from build123d import *

# Parameters (mm, degrees)
PAD_DEPTH = 5
FILLET_R  = 1


with BuildPart() as part:
    # Sketch → Pad (new body)
    with BuildSketch(Plane.XZ):
        with BuildLine():
            Line((-8, 5.95), (-8, -6.95))
            Line((-8, -6.95), (-5.7, -6.95))
            Line((-5.7, -6.95), (-5.7, -10.75))
            Line((-5.7, -10.75), (-8.5, -10.75))
            ThreePointArc((-10.5, -8.75), (-9.914214, -10.164214), (-8.5, -10.75))
            Line((-10.5, -8.75), (-10.5, 7.45))
            ThreePointArc((-8.5, 9.45), (-9.914214, 8.864214), (-10.5, 7.45))
            Line((-8.5, 9.45), (8.5, 9.45))
            ThreePointArc((10.5, 7.45), (9.914214, 8.864214), (8.5, 9.45))
            Line((10.5, 7.45), (10.5, -8.75))
            ThreePointArc((8.5, -10.75), (9.914214, -10.164214), (10.5, -8.75))
            Line((8.5, -10.75), (5.7, -10.75))
            Line((5.7, -10.75), (5.7, -6.95))
            Line((5.7, -6.95), (8, -6.95))
            Line((8, -6.95), (8, 5.95))
            ThreePointArc((8, 5.95), (7.707107, 6.657107), (7, 6.95))
            Line((7, 6.95), (-7, 6.95))
            ThreePointArc((-7, 6.95), (-7.707107, 6.657107), (-8, 5.95))
        make_face()
    extrude(amount=PAD_DEPTH)

    # Fillet
    fillet_edges = [part.edges().sort_by_distance(p)[0] for p in [
        (-6.85, -5, -6.95),
        (-8, -5, -0.5),
        (-5.7, -2.5, -6.95),
        (-5.7, -5, -8.85),
        (-5.7, -2.5, -10.75),
        (-10.5, -5, -0.65),
        (-8, 0, -0.5),
        (-6.85, 0, -6.95),
        (-5.7, 0, -8.85),
        (0, 0, 9.45),
        (5.7, -5, -8.85),
        (5.7, -2.5, -10.75),
        (5.7, 0, -8.85),
        (5.7, -2.5, -6.95),
        (6.85, -5, -6.95),
        (7.1, -5, -10.75),
        (10.5, -5, -0.65),
        (8, -5, -0.5),
        (8, 0, -0.5),
        (-10.5, 0, -0.65),
        (0, -5, 9.45),
        (10.5, 0, -0.65),
        (6.85, 0, -6.95),
    ]]
    fillet(fillet_edges, radius=FILLET_R)


solid = part.part
Design review of the part built by this model. Coordinates are the model's own, in mm. A direction names the side the tool comes from. Round coordinates to 2 decimals unless told otherwise and drop trailing zeros. Write each loop counter-clockwise with the first axis right and the second up, starting at its lowest first coordinate (ties: lowest second). Pieces come first, ordered by that corner, then holes. Notation, with made-up numbers: (55.5, 66) - (111.5, 66) arc R20 cw to (111.5, 72) - close; hole circle Ø2 at (48.25, 0.5). An arc over 180 degrees is marked (long way). Return JSON: item names as keys, results as strings. Group by question number.
Item 1: We need section D-D on z = -7.5. Write out the cut boundary in (x, y).
Item 2: We need section B-B on y = -1.65. Write out the cut boundary in (x, z).
Item 3: Insertion check: P1, Ø0.9, axis at x = 1.5, y = -2, coming from the -Z side; P2, Ø0.9, axis at y = -2, z = -9, coming from the +X side; P3, Ø2, axis at x = -6.5, z = -6.5, coming from the -Y side. Each pin has a flat end and moves straight along its axis. Give the tip position at first contact, or say it passes through.
Item 4: We need section A-A on z = -1. Write out the cut boundary in (x, y).
Item 5: We need section C-C on x = 2.5. Write out the cut boundary in (y, z), and give its area (3 significant figures).
Item 6: For probe 1 along X at (y, z) = (-3.4, 5.75); probe 2 along X at (y, z) = (-1.15, -8.5); probe 3 along Z at (x, y) = (-3.25, -2.1), list the stretches that pass through material, from the lowest coordinate up. Write a range as [from, to].
Item 7: Machinability: for faces 1 (the face through (-0.098, -0.301, 7.235)), 2 (the face through (-7.699, -2.479, 6.665)), 3 (the face through (8.285, -4.699, -0.903)), 4 (the face through (-5.985, -4.699, -8.863)), which of the approach directions +Z, -Z, +X, -X, +Y, -Y give a long, thin tool a straight path to every point of the face, cutting with its end or side? Answer none if there is none.
Item 8: The part is to be moulded in two halves that separate along Z. For faces 5 (the face through (10.215, -4.699, -0.763)), 6 (the face through (5.985, -2.521, -7.251)), 7 (the face through (7.587, -0.301, -10.465)), say which applies: pulls with the +Z half, pulls with the -Z half, needs draft (parallel to the pull), parting line crosses it, or undercut.
Model answer:
{
 "1": {"outline": "(-10.5, -4) arc R1 ccw to (-9.5, -5) - (-9, -5) arc R1 ccw to (-8.55, -4.89) - (-6.7, -4.89) arc R0.89 ccw to (-5.81, -4) - (-5.81, -1) arc R0.89 ccw to (-6.7, -0.11) - (-8.55, -0.11) arc R1 ccw to (-9, 0) - (-9.5, 0) arc R1 ccw to (-10.5, -1) - close; (5.81, -4) arc R0.89 ccw to (6.7, -4.89) - (8.55, -4.89) arc R1 ccw to (9, -5) - (9.5, -5) arc R1 ccw to (10.5, -4) - (10.5, -1) arc R1 ccw to (9.5, 0) - (9, 0) arc R1 ccw to (8.55, -0.11) - (6.7, -0.11) arc R0.89 ccw to (5.81, -1) - close"},
 "2": {"outline": "(-10.5, -8.75) arc R2 ccw to (-8.5, -10.75) - (-6.7, -10.75) arc R1 ccw to (-5.7, -9.75) - (-5.7, -7.95) arc R1 ccw to (-6.7, -6.95) - (-8, -6.95) - (-8, 5.95) arc R1 cw to (-7, 6.95) - (7, 6.95) arc R1 cw to (8, 5.95) - (8, -6.95) - (6.7, -6.95) arc R1 ccw to (5.7, -7.95) - (5.7, -9.75) arc R1 ccw to (6.7, -10.75) - (8.5, -10.75) arc R2 ccw to (10.5, -8.75) - (10.5, 7.45) arc R2 ccw to (8.5, 9.45) - (-8.5, 9.45) arc R2 ccw to (-10.5, 7.45) - close"},
 "3": {"P1": "stops at z = 6.95", "P2": "stops at x = 10.5", "P3": "stops at y = -4.89"},
 "4": {"outline": "(-10.5, -4) arc R1 ccw to (-9.5, -5) - (-9, -5) arc R1 ccw to (-8, -4) - (-8, -1) arc R1 ccw to (-9, 0) - (-9.5, 0) arc R1 ccw to (-10.5, -1) - close; (8, -4) arc R1 ccw to (9, -5) - (9.5, -5) arc R1 ccw to (10.5, -4) - (10.5, -1) arc R1 ccw to (9.5, 0) - (9, 0) arc R1 ccw to (8, -1) - close"},
 "5": {"outline": "(-5, 7.95) arc R1 ccw to (-4, 6.95) - (-1, 6.95) arc R1 ccw to (0, 7.95) - (0, 8.45) arc R1 ccw to (-1, 9.45) - (-4, 9.45) arc R1 ccw to (-5, 8.45) - close", "area": "11.6 mm²"},
 "6": {"probe 1": "x = [-10.5, -8], [8, 10.5]", "probe 2": "x = [-10.5, -5.7], [5.7, 10.5]", "probe 3": "z = [6.95, 9.45]"},
 "7": {"face 1": "+Y", "face 2": "+Y, -Y", "face 3": "-Y", "face 4": "-Z, -Y"},
 "8": {"face 5": "needs draft", "face 6": "undercut", "face 7": "pulls with the -Z half"}
}
